from build123d import *

# Parameters (mm, degrees)
F1_DEPTH = 500
F2_SIZE  = 1
F3_SIZE  = 1
F4_SIZE  = 1
F5_D     = 4
F6_D     = 4
F7_D     = 4
F8_D     = 4
F9_D     = 6.25


with BuildPart() as f1:
    # F0 (on Front) → F1 (new body)
    with BuildSketch(Plane.XZ):
        with BuildLine():
            Line((12.5, -12.5), (12.5, -3.25))
            Line((12.5, -3.25), (10.8, -3.25))
            Line((10.8, -3.25), (10.8, -5.4))
            Line((10.8, -5.4), (6.25, -5.4))
            ThreePointArc((6.25, -5.4), (5.4, 0), (6.25, 5.4))
            Line((6.25, 5.4), (10.8, 5.4))
            Line((10.8, 5.4), (10.8, 3.25))
            Line((10.8, 3.25), (12.5, 3.25))
            Line((12.5, 3.25), (12.5, 12.5))
            Line((12.5, 12.5), (3.25, 12.5))
            Line((3.25, 12.5), (3.25, 10.8))
            Line((3.25, 10.8), (5.4, 10.8))
            Line((5.4, 10.8), (5.4, 6.25))
            ThreePointArc((5.4, 6.25), (0, 5.4), (-5.4, 6.25))
            Line((-5.4, 6.25), (-5.4, 10.8))
            Line((-5.4, 10.8), (-3.25, 10.8))
            Line((-3.25, 10.8), (-3.25, 12.5))
            Line((-3.25, 12.5), (-12.5, 12.5))
            Line((-12.5, 12.5), (-12.5, 3.25))
            Line((-12.5, 3.25), (-10.8, 3.25))
            Line((-10.8, 3.25), (-10.8, 5.4))
            Line((-10.8, 5.4), (-6.25, 5.4))
            ThreePointArc((-6.25, 5.4), (-5.4, 0), (-6.25, -5.4))
            Line((-6.25, -5.4), (-10.8, -5.4))
            Line((-10.8, -5.4), (-10.8, -3.25))
            Line((-10.8, -3.25), (-12.5, -3.25))
            Line((-12.5, -3.25), (-12.5, -12.5))
            Line((-12.5, -12.5), (-3.25, -12.5))
            Line((-3.25, -12.5), (-3.25, -10.8))
            Line((-3.25, -10.8), (-5.4, -10.8))
            Line((-5.4, -10.8), (-5.4, -6.25))
            ThreePointArc((-5.4, -6.25), (0, -5.4), (5.4, -6.25))
            Line((5.4, -6.25), (5.4, -10.8))
            Line((5.4, -10.8), (3.25, -10.8))
            Line((3.25, -10.8), (3.25, -12.5))
            Line((3.25, -12.5), (12.5, -12.5))
        make_face()
    extrude(amount=F1_DEPTH)

    # F2
    f2_edges = [f1.edges().sort_by_distance(p)[0] for p in [
        (-12.5, -250, 12.5),
    ]]
    chamfer(f2_edges, length=F2_SIZE)

    # F3
    f3_edges = [f1.edges().sort_by_distance(p)[0] for p in [
        (12.5, -250, 12.5),
        (12.5, -250, -12.5),
        (-12.5, -250, -12.5),
    ]]
    chamfer(f3_edges, length=F3_SIZE)

    # F4
    f4_edges = [f1.edges().sort_by_distance(p)[0] for p in [
        (3.25, -250, 10.8),
        (10.8, -250, 3.25),
        (10.8, -250, -3.25),
        (3.25, -250, -10.8),
        (-3.25, -250, -10.8),
        (-10.8, -250, -3.25),
        (-3.25, -250, 10.8),
        (-10.8, -250, 3.25),
    ]]
    chamfer(f4_edges, length=F4_SIZE)

    # F5 (through all)
    with Locations(Plane(origin=(0, 0, 0), x_dir=(1, 0, 0), z_dir=(0, 1, 0))):
        with Locations((8.95, -8.95)):
            Hole(F5_D / 2)

    # F6 (through all)
    with Locations(Plane(origin=(0, 0, 0), x_dir=(1, 0, 0), z_dir=(0, 1, 0))):
        with Locations((8.95, 8.95)):
            Hole(F6_D / 2)

    # F7 (through all)
    with Locations(Plane(origin=(0, 0, 0), x_dir=(1, 0, 0), z_dir=(0, 1, 0))):
        with Locations((-8.95, -8.95)):
            Hole(F7_D / 2)

    # F8 (through all)
    with Locations(Plane(origin=(0, 0, 0), x_dir=(1, 0, 0), z_dir=(0, 1, 0))):
        with Locations((-8.95, 8.95)):
            Hole(F8_D / 2)

    # F9 (through all)
    with Locations(Plane(origin=(0, 0, 0), x_dir=(1, 0, 0), z_dir=(0, 1, 0))):
        with Locations((0, 0)):
            Hole(F9_D / 2)


solid = f1.part
For this review, take the finished solid that the model builds, in its own axes (mm). A direction names the side the tool comes from. Round coordinates to 2 decimals unless told otherwise and drop trailing zeros. Put each result on its own line as item: value.
Q1. Machinability: for faces 4 (the cylindrical face through (5.4, -246.5, -0.1)), 5 (the flat face through (7, -246, -12.5)), which of the approach directions +Z, -Z, +X, -X, +Y, -Y give a long, thin tool a straight path to every point of the face, cutting with its end or side? Answer none if there is none.
Check result:
face 4: +Y, -Y
face 5: -Z, +X, -X, +Y, -Y
Q2. Mouldability with a two-part tool opening along X and no side actions: class faces 1 (the flat face through (12.5, -246, -7)), 2 (the flat face through (3, -500, -3)), 3 (the cylindrical face through (0.1, -246.5, 5.4)) as pulls with the +X half, pulls with the -X half, needs draft (parallel to the pull), parting line crosses it, or undercut.
Check result:
face 1: pulls with the +X half
face 2: needs draft
face 3: undercut
Q3. For probe 1 along Z at (x, y) = (9, -177.5); probe 2 along Z at (x, y) = (4, -298), list the stretches that pass through material, from the lowest coordinate up. Write a range as [from, to].
Check result:
probe 1: [-12.5, -10.95], [-6.95, -5.4], [5.4, 6.95], [10.95, 12.5]
probe 2: [-12.5, -11.05], [-5.86, 5.86], [11.05, 12.5]
Q4. Insertion check: pin 1 Ø1 at (x, y) = (-1, -210.5) entering from -Z; pin 2 Ø1.5 at (x, y) = (0.5, -410.5) entering from -Z. Each pin has a flat end and moves straight along its axis. Give the tip position at first contact, or say it passes through.
Check result:
pin 1: z = -5.46
pin 2: z = -5.44
Q5. Add section A-A on y = -459.5. State how many separate pieces and enclosed holes the cut face has, plus the area to 3 significant figures.
Check result:
separate pieces: 1
enclosed holes: 5
area: 273 mm2
